```python
from build123d import *

# Parameters (mm, degrees)
SKETCH1_R               = 10
BOSS_EXTRUDE1_DEPTH     = 81.5
CUT_EXTRUDE1_DEPTH      = 25
CUT_EXTRUDE1_DEPTH_BACK = 19
SKETCH3_R               = 2
SKETCH4_R               = 15
BOSS_EXTRUDE2_DEPTH     = 5
SCALE1_SCALE            = 0.5


with BuildPart() as part:
    # Sketch1 → Boss-Extrude1 (new body)
    with BuildSketch(Plane(origin=(0, 0, 0), x_dir=(0, 0, -1), z_dir=(1, 0, 0))):
        Circle(SKETCH1_R)
    extrude(amount=BOSS_EXTRUDE1_DEPTH)

    # Sketch3 → Cut-Extrude1 (cut, two sides: drawn at the far end of the back side and taken through both)
    with BuildSketch(Plane.XY.offset(-CUT_EXTRUDE1_DEPTH_BACK)):
        with Locations((78, 0)):
            Circle(SKETCH3_R)
    extrude(amount=CUT_EXTRUDE1_DEPTH + CUT_EXTRUDE1_DEPTH_BACK, mode=Mode.SUBTRACT)

    # Sketch4 → Boss-Extrude2 (add)
    with BuildSketch(Plane.ZY):
        Circle(SKETCH4_R)
    extrude(amount=-BOSS_EXTRUDE2_DEPTH)


with BuildPart() as part_1:
    # Scale1: scaled about (0, 0, 0)
    add(part.part.scale(SCALE1_SCALE))


solid = part_1.part
```
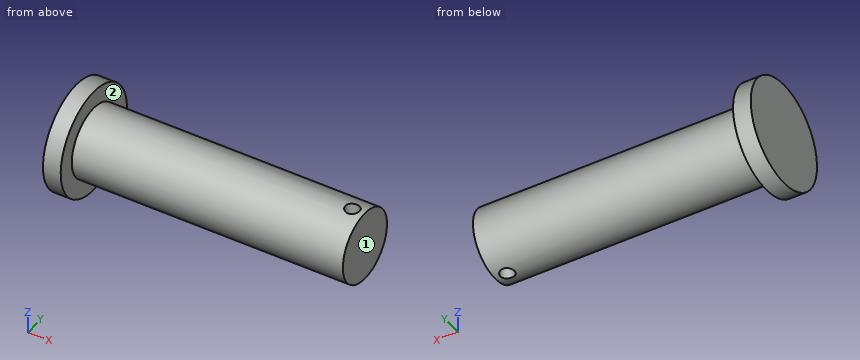
Can you work these out from the model? Positions are in its coordinate system, mm. Face numbers are marked on the shaded views. A direction names the side the tool comes from. Coordinates: 2 decimals unless noted, no trailing zeros. Order: outer loops, then holes, each group sorted by start corner. A loop starts at its lowest first (then second) coordinate and runs counter-clockwise, first axis right, second up. Notation, with made-up numbers: (-4.75, 40) -> (44.25, 40) arc R14 ccw to (44.25, 53) -> close; hole circle Ø10 at (21, 67.5). An arc over 180 degrees is marked (long way). Write each question's results on one line, items separated by ' | '.
Item 1: I want a section at B-B, the plane y = 0. Write out the boundary of the cut face in (x, z).
Results are:
outline: (0, -7.5) -> (2.5, -7.5) -> (2.5, -5) -> (38, -5) -> (38, 5) -> (2.5, 5) -> (2.5, 7.5) -> (0, 7.5) -> close; (40, -5) -> (40.75, -5) -> (40.75, 5) -> (40, 5) -> close
Item 2: Which directions (+Z, -Z, +X, -X, +Y, -Y) give clear straight access to the entire face, cutting with the end or side of a thin tool? Please do the marked faces 1 and 2.
Results are:
face 1: +Z, -Z, +X, +Y, -Y | face 2: +X
Item 3: If I drill on line 1 along X through (y, z) = (0, 1); line 2 along Z through (x, y) = (19.5, 0.25), over which ranges is the centre line in solid material (lowest first)?
Results are:
line 1: 0 to 38, 40 to 40.75 | line 2: -4.99 to 4.99
Item 4: I want a section at D-D, the plane z = 1.75. Write out the boundary of the cut face in (x, y).
Results are:
outline: (0, -7.29) -> (2.5, -7.29) -> (2.5, -4.68) -> (40.75, -4.68) -> (40.75, 4.68) -> (2.5, 4.68) -> (2.5, 7.29) -> (0, 7.29) -> close; hole circle Ø2 at (39, 0)
Item 5: I'm going to push flat-ended pins straight in: pin 1 Ø4 at (x, z) = (20.5, -3.5) entering from +Y; pin 2 Ø1.5 at (x, y) = (32.5, 5) entering from +Z; pin 3 Ø2 at (x, z) = (29, -1) entering from +Y. Where does each tip first touch, or does it pass through?
Results are:
pin 1: y = 4.77 | pin 2: z = 2.63 | pin 3: y = 5
Item 6: I want a section at C-C, the plane x = 39. Write out the boundary of the cut face in (y, z).
Results are:
outline: (-1, -4.9) -> (-1, 4.9) arc R5 ccw to start; (1, -4.9) arc R5 ccw to (1, 4.9) -> close
Item 7: I want a section at A-A, the plane z = 0. Write out the boundary of the cut face in (x, y), then the cut area to 3 significant figures.
Results are:
outline: (0, -7.5) -> (2.5, -7.5) -> (2.5, -5) -> (40.75, -5) -> (40.75, 5) -> (2.5, 5) -> (2.5, 7.5) -> (0, 7.5) -> close; hole circle Ø2 at (39, 0) | area: 417 mm²
